from build123d import *

# Parameters (mm, degrees)
BOSS_EXTRUDE1_DEPTH = 38
BOSS_EXTRUDE2_DEPTH = 10
FILLET1_R           = 5
SKETCH3_R           = 9
CUT_EXTRUDE1_DEPTH  = 5
SKETCH5_R           = 9
BOSS_EXTRUDE3_DEPTH = 0.5
SKETCH6_R           = 3
CUT_EXTRUDE2_DEPTH  = 2.5


with BuildPart() as part:
    # Sketch1 → Boss-Extrude1 (new body)
    with BuildSketch(Plane(origin=(0, 0, 0), x_dir=(1, 0, 0), z_dir=(0, 1, 0))):
        Polygon((-142, 0), (142, 0), (107, 62), (-107, 62), align=None)
    extrude(amount=BOSS_EXTRUDE1_DEPTH)

    # Sketch2 → Boss-Extrude2 (add)
    with BuildSketch(Plane.XZ):
        with BuildLine():
            ThreePointArc((8.5, -31), (0, -35.75), (-8.5, -31))
            ThreePointArc((-8.5, -31), (0, -26.25), (8.5, -31))
        make_face()
    extrude(amount=BOSS_EXTRUDE2_DEPTH)

    # Fillet1
    fillet1_edges = [part.edges().sort_by_distance(p)[0] for p in [
        (124.5, 38, -31),
        (0, 38, -62),
        (-124.5, 38, -31),
        (0, 0, -62),
        (124.5, 0, -31),
        (0, 0, 0),
        (-124.5, 0, -31),
        (0, 38, 0),
        (-107, 19, -62),
        (107, 19, -62),
        (142, 19, 0),
        (-142, 19, 0),
    ]]
    fillet(fillet1_edges, radius=FILLET1_R)

    # Sketch3 → Cut-Extrude1 (cut)
    with BuildSketch(Plane.XY):
        with Locations((12.5, 19)):
            Circle(SKETCH3_R)
        with Locations((-12.5, 19)):
            Circle(SKETCH3_R)
        with Locations((-62.5, 19)):
            Circle(SKETCH3_R)
    extrude(amount=-CUT_EXTRUDE1_DEPTH, mode=Mode.SUBTRACT)

    # Sketch5 → Boss-Extrude3 (add, symmetric)
    with BuildSketch(Plane.XY):
        with Locations((-12.5, 19)):
            Circle(SKETCH5_R)
        with Locations((12.5, 19)):
            Circle(SKETCH5_R)
        with Locations((-62.5, 19)):
            Circle(SKETCH5_R)
    extrude(amount=BOSS_EXTRUDE3_DEPTH, both=True)

    # Sketch6 → Cut-Extrude2 (cut)
    with BuildSketch(Plane.XZ):
        with Locations((-97, -17.5)):
            Circle(SKETCH6_R)
        with Locations((97, -17.5)):
            Circle(SKETCH6_R)
    extrude(amount=-CUT_EXTRUDE2_DEPTH, mode=Mode.SUBTRACT)


solid = part.part
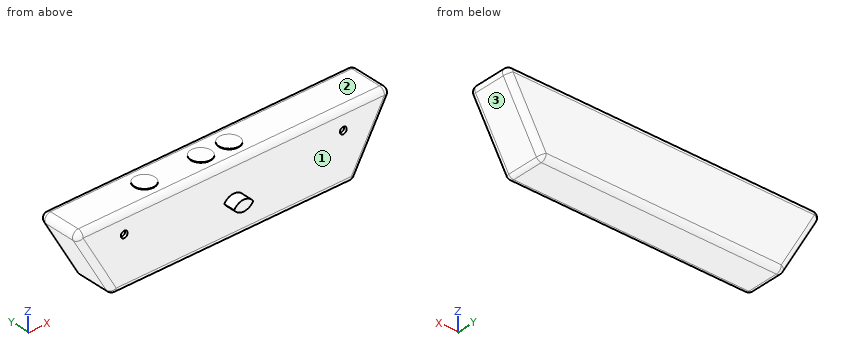
Design review of the part built by this model. Coordinates are the model's own, in mm. Face numbers are marked on the shaded views. Coordinates: 2 decimals unless noted, no trailing zeros. Loops run counter-clockwise (first coordinate to the right, second up) from the corner with the lowest first, then second, coordinate; pieces in that order, holes last. Notation, with made-up numbers: M 81,71.5 L 117,71.5 A15 cw 117,80.5 Z; hole C 67,-0.5 d6. An arc over 180 degrees is marked long. Use one line per item in the form item = value.
(1) Draft analysis for pull direction X (two halves, no side actions). For the marked faces 1, 2 and 3, state which applies: pulls with the +X half, pulls with the -X half, needs draft (parallel to the pull), parting line crosses it, or undercut.
Return value:
face_1 = needs draft
face_2 = undercut
face_3 = pulls with the +X half
(2) For line 1 along Y through (x, z) = (-60.5, -27.5); line 2 along Z through (x, y) = (-12.5, 21); line 3 along Y through (x, z) = (-62.5, -3.75), list the stretches that pass through material, from the lowest coordinate up. Write a range as from..to.
Return value:
line_1 = 0..38
line_2 = -62..-5, -0.5..0.5
line_3 = 0.16..10, 28..37.84
(3) Consider section B-B (y = 19). Give the number of separate pieces and of enclosed holes in the cut face, and give its area (3 significant figures).
Return value:
separate_pieces = 1
enclosed_holes = 3
area = 15,200 mm2
(4) Consider section A-A (x = -62.5). Write out the cut boundary in (y, z).
Return value:
outline = M 0,-57 A5 ccw 5,-62 L 33,-62 A5 ccw 38,-57 L 38,-5 A5 ccw 33,0 L 28,0 L 28,0.5 L 10,0.5 L 10,0 L 5,0 A5 ccw 0,-5 Z; hole M 10,-5 L 28,-5 L 28,-0.5 L 10,-0.5 Z
(5) Clearance check with flat-ended pins moving along their axes: P1, Ø10, axis at x = 73.5, y = 32, coming from the +Z side; P2, Ø6.5, axis at x = -98, z = -17.5, coming from the -Y side; P3, Ø3, axis at y = 2, z = -33.5, coming from the -X side. State where each tip first meets the part, or that it passes through.
Return value:
P1 = 0
P2 = 0
P3 = -123.24
(6) Consider section D-D (x = 19). Write out the cut boundary in (y, z).
Return value:
outline = M 0,-57 A5 ccw 5,-62 L 33,-62 A5 ccw 38,-57 L 38,-5 A5 ccw 33,0 L 25.22,0 L 25.22,0.5 L 12.78,0.5 L 12.78,0 L 5,0 A5 ccw 0,-5 Z; hole M 12.78,-5 L 25.22,-5 L 25.22,-0.5 L 12.78,-0.5 Z
(7) Consider section C-C (x = -97). Write out the cut boundary in (y, z), and give its area (3 significant figures).
Return value:
outline = M 0,-57 A5 ccw 5,-62 L 33,-62 A5 ccw 38,-57 L 38,-5 A5 ccw 33,0 L 5,0 A5 ccw 0,-5 L 0,-14.5 L 2.5,-14.5 L 2.5,-20.5 L 0,-20.5 Z
area = 2,320 mm2
